```python
from build123d import *

# Parameters (mm, degrees)
F0_W     = 40
F0_H     = 40
F0_R     = 3
F0_R_2   = 18
F1_DEPTH = 5
F2_DEPTH = 8.5
F3_R     = 5
F4_R     = 1.99999
F0_R_3   = 1.96412235
F5_DEPTH = 2.5


# Not quite as in the source:
# - a fillet or chamfer is up to 0.001 mm smaller than in the source, because OpenCascade refuses the exact size


with BuildPart() as f1:
    # F0 (on Top) → F1 (new body)
    with BuildSketch(Plane.XY):
        Rectangle(F0_W, F0_H)
        with Locations((-16, 15.8712012513)):
            Circle(F0_R, mode=Mode.SUBTRACT)
        Circle(F0_R_2, mode=Mode.SUBTRACT)
        with Locations((16, 15.8712012513)):
            Circle(F0_R, mode=Mode.SUBTRACT)
    extrude(amount=F1_DEPTH)

    # F0 (on Top) → F2 (join)
    with BuildSketch(Plane.XY):
        with Locations((-16, 15.8712012513)):
            Circle(F0_R)
        with Locations((16, 15.8712012513)):
            Circle(F0_R)
    extrude(amount=F2_DEPTH)

    # F3
    f3_edges = [f1.edges().sort_by_distance(p)[0] for p in [
        (-20, -20, 2.5),
        (-20, 20, 2.5),
        (20, -20, 2.5),
        (20, 20, 2.5),
    ]]
    fillet(f3_edges, radius=F3_R)

    # F4 (radius 2 in the source; OpenCascade refuses exactly that, so slightly less here)
    f4_edges = [f1.edges().sort_by_distance(p)[0] for p in [
        (20, 0, 0),
    ]]
    fillet(f4_edges, radius=F4_R)

    # F0 (on Top) → F5 (join)
    with BuildSketch(Plane.XY):
        Circle(F0_R_2)
        with BuildLine():
            ThreePointArc((15.8087915907, 2.4661931072), (15.952126276, 1.236797184), (16, 0))
            ThreePointArc((16, 0), (13.1965480074, -9.0471609187), (5.7686099139, -14.9239116743))
            ThreePointArc((5.7686099139, -14.9239116743), (0, -16), (-5.7686099139, -14.9239116743))
            ThreePointArc((-5.7686099139, -14.9239116743), (-13.8564064606, -8), (-15.8087915907, 2.4661931072))
            ThreePointArc((-15.8087915907, 2.4661931072), (-13.8564064606, 8), (-10.0401816768, 12.4577185671))
            ThreePointArc((-10.0401816768, 12.4577185671), (0, 16), (10.0401816768, 12.4577185671))
            ThreePointArc((10.0401816768, 12.4577185671), (13.8564064606, 8), (15.8087915907, 2.4661931072))
        make_face(mode=Mode.SUBTRACT)
        with BuildLine():
            ThreePointArc((3.96412235, 0), (3.9439266403, 0.3996356611), (3.8835452903, 0.795199336))
            ThreePointArc((3.8835452903, 0.795199336), (3.4330306588, 1.982061175), (2.6304354712, 2.9656492102))
            ThreePointArc((2.6304354712, 2.9656492102), (0, 3.96412235), (-2.6304354712, 2.9656492102))
            ThreePointArc((-2.6304354712, 2.9656492102), (-3.4330306588, 1.982061175), (-3.8835452903, 0.795199336))
            ThreePointArc((-3.8835452903, 0.795199336), (-3.4330306588, -1.982061175), (-1.2531098191, -3.7608485461))
            ThreePointArc((-1.2531098191, -3.7608485461), (0, -3.96412235), (1.2531098191, -3.7608485461))
            ThreePointArc((1.2531098191, -3.7608485461), (3.2157228306, -2.3180579549), (3.96412235, 0))
        make_face()
        Circle(F0_R_3, mode=Mode.SUBTRACT)
        with BuildLine():
            ThreePointArc((-5.7686099139, -14.9239116743), (0, -16), (5.7686099139, -14.9239116743))
            Line((5.7686099139, -14.9239116743), (1.2531098191, -3.7608485461))
            ThreePointArc((1.2531098191, -3.7608485461), (0, -3.96412235), (-1.2531098191, -3.7608485461))
            Line((-1.2531098191, -3.7608485461), (-5.7686099139, -14.9239116743))
        make_face()
        with BuildLine():
            Line((3.8835452903, 0.795199336), (15.8087915907, 2.4661931072))
            ThreePointArc((15.8087915907, 2.4661931072), (13.8564064606, 8), (10.0401816768, 12.4577185671))
            Line((10.0401816768, 12.4577185671), (2.6304354712, 2.9656492102))
            ThreePointArc((2.6304354712, 2.9656492102), (3.4330306588, 1.982061175), (3.8835452903, 0.795199336))
        make_face()
        with BuildLine():
            Line((-2.6304354712, 2.9656492102), (-10.0401816768, 12.4577185671))
            ThreePointArc((-10.0401816768, 12.4577185671), (-13.8564064606, 8), (-15.8087915907, 2.4661931072))
            Line((-15.8087915907, 2.4661931072), (-3.8835452903, 0.795199336))
            ThreePointArc((-3.8835452903, 0.795199336), (-3.4330306588, 1.982061175), (-2.6304354712, 2.9656492102))
        make_face()
    extrude(amount=F5_DEPTH)


solid = f1.part
```
The model under review builds one solid part; all positions refer to its coordinate system, in mm. A direction names the side the tool comes from. Coordinates: 2 decimals unless noted, no trailing zeros. Write each loop counter-clockwise with the first axis right and the second up, starting at its lowest first coordinate (ties: lowest second). Pieces come first, ordered by that corner, then holes.
1) We need section B-B on x = 0. State the section outline as (y, z) points, then the cut area to 3 significant figures.
2) We need section D-D on y = -9. State the section outline as (x, z) points.
3) Clearance check with flat-ended pins moving along their axes: pin 1 Ø12 at (x, y) = (-0.5, -11) entering from +Z; pin 2 Ø2 at (x, y) = (13.5, 10.5) entering from +Z. State where each tip first meets the part, or that it passes through.
4) We need section C-C on y = 6.5. State the section outline as (x, z) points.
5) To check wall thickness, follow probe 1 along Y at (x, z) = (0, 3.9); probe 2 along Y at (x, z) = (0, 0.7); probe 3 along Y at (x, z) = (3, 0.75). State the ranges of each line that lie inside material, in increasing order.
6) Machinability: for faces 4 (the face through (6.39, 7.78, 1.23)), 5 (the face through (0, -4, 2.5)), 6 (the face through (-19.43, -0.21, 0.6)), which of the approach directions +Z, -Z, +X, -X, +Y, -Y give a long, thin tool a straight path to every point of the face, cutting with its end or side? Answer none if there is none.
7) We need section A-A on z = 3.5. State the section outline as (x, y) points.
8) The part is to be moulded in two halves that separate along Y. For faces 1 (the face through (0, -4, 0)), 2 (the face through (-3.45, -1.95, 1.23)), 3 (the face through (18, -19, 4)), say which applies: pulls with the +Y half, pulls with the -Y half, needs draft (parallel to the pull), parting line crosses it, or undercut.
Answer list:
1. outline: (-20, 2) arc R2 ccw to (-18, 0) - (-1.96, 0) - (-1.96, 2.5) - (-18, 2.5) - (-18, 5) - (-20, 5) - close; (1.96, 0) - (3.96, 0) - (3.96, 2.5) - (1.96, 2.5) - close; (16, 0) - (18, 0) arc R2 ccw to (20, 2) - (20, 5) - (18, 5) - (18, 2.5) - (16, 2.5) - close
1. area: 68.4 mm2
2. outline: (-20, 2) arc R2 ccw to (-18, 0) - (-13.23, 0) - (-13.23, 2.5) - (-15.59, 2.5) - (-15.59, 5) - (-20, 5) - close; (-3.37, 0) - (3.37, 0) - (3.37, 2.5) - (-3.37, 2.5) - close; (13.23, 0) - (18, 0) arc R2 ccw to (20, 2) - (20, 5) - (15.59, 5) - (15.59, 2.5) - (13.23, 2.5) - close
3. pin 1: stops at z = 2.5
3. pin 2: stops at z = 5
4. outline: (-20, 2) arc R2 ccw to (-18, 0) - (-5.39, 0) - (-5.39, 2.5) - (-16.79, 2.5) - (-16.79, 5) - (-20, 5) - close; (5.39, 0) - (18, 0) arc R2 ccw to (20, 2) - (20, 5) - (16.79, 5) - (16.79, 2.5) - (5.39, 2.5) - close
5. probe 1: y = -20 to -18, 18 to 20
5. probe 2: y = -19.52 to -1.96, 1.96 to 3.96, 16 to 19.52
5. probe 3: y = -19.56 to -8.08, -2.59 to 3.44, 15.72 to 19.56
6. face 4: +Z, -Z
6. face 5: +Z
6. face 6: -Z, -X, +Y, -Y
7. outline: (-20, -15) arc R5 ccw to (-15, -20) - (15, -20) arc R5 ccw to (20, -15) - (20, 15) arc R5 ccw to (15, 20) - (-15, 20) arc R5 ccw to (-20, 15) - close; hole circle Ø36 at (0, 0)
8. face 1: needs draft
8. face 2: undercut
8. face 3: pulls with the -Y half
